from build123d import *
from build123d.topology import SkipClean

# Parameters (mm, degrees)
SKETCH2_R               = 50.165
BOSS_EXTRUDE1_DEPTH     = 38.862
SKETCH3_R               = 14.986
BOSS_EXTRUDE2_DEPTH     = 3.556
BOSS_EXTRUDE3_START     = 2.54
SKETCH4_R               = 50.165
SKETCH4_R_2             = 43.18
BOSS_EXTRUDE3_DEPTH     = 2.54
SKETCH5_R               = 8.89
CUT_EXTRUDE1_DEPTH      = 81.890725637
CIRPATTERN1_COUNT       = 4
CUT_EXTRUDE2_DEPTH      = 83.657977074
CUT_EXTRUDE2_DEPTH_BACK = 83.657977074
SKETCH6_R               = 2.54
SKETCH7_R               = 10.033
SKETCH7_R_2             = 8.001
BOSS_EXTRUDE4_DEPTH     = 1.016
SKETCH8_R               = 4.953
SKETCH8_R_2             = 2.54
BOSS_EXTRUDE5_DEPTH     = 1.016
CHAMFER1_SIZE           = 0.254
FILLET1_R               = 0.254
CHAMFER2_SIZE           = 1.27
CHAMFER3_SIZE           = 1.27
CHAMFER4_SIZE           = 0.254


with BuildPart() as part:
    # Sketch2 → Boss-Extrude1 (new body)
    with BuildSketch(Plane.XY):
        with Locations(Location((0, 0, 0), (0, 0, 180))):
            Circle(SKETCH2_R)
    extrude(amount=BOSS_EXTRUDE1_DEPTH)

    # Sketch3 → Boss-Extrude2 (add)
    with BuildSketch(Plane(origin=(0, 0, 0), x_dir=(-1, 0, 0), z_dir=(0, 0, -1))):
        with Locations(Location((0, 0, 0), (0, 0, 180))):
            Circle(SKETCH3_R)
    boss_extrude2 = extrude(amount=BOSS_EXTRUDE2_DEPTH)

    # Sketch4 → Boss-Extrude3 (add)
    with BuildSketch(Plane(origin=(0, 0, 0), x_dir=(-1, 0, 0), z_dir=(0, 0, -1)).offset(BOSS_EXTRUDE3_START)):
        Circle(SKETCH4_R)
        Circle(SKETCH4_R_2, mode=Mode.SUBTRACT)
    boss_extrude3 = extrude(amount=-BOSS_EXTRUDE3_DEPTH)

    # Sketch5 → Cut-Extrude1 (cut, through all)
    with BuildSketch(Plane(origin=(0, 0, 0), x_dir=(-1, 0, 0), z_dir=(0, 0, -1))):
        with Locations((31.75, 0)):
            Circle(SKETCH5_R)
    cut_extrude1 = extrude(amount=-CUT_EXTRUDE1_DEPTH, mode=Mode.SUBTRACT)

    # CirPattern1: Cut-Extrude1 ×4 about axis
    cirpattern1_axis = Axis((0, 0, 0), (0, 0, 1))
    for i in range(1, CIRPATTERN1_COUNT):
        add(cut_extrude1.rotate(cirpattern1_axis, i * 360 / CIRPATTERN1_COUNT), mode=Mode.SUBTRACT)

    # Mirror1: Boss-Extrude3 across plane
    add(boss_extrude3.mirror(Plane(origin=(0, 0, 19.431), x_dir=(1, 0, 0), z_dir=(0, 0, -1))))

    # Mirror2: Boss-Extrude2 across plane
    add(boss_extrude2.mirror(Plane(origin=(0, 0, 19.431), x_dir=(1, 0, 0), z_dir=(0, 0, -1))))

    # Sketch6 → Cut-Extrude2 (cut, two sides: drawn at the far end of the back side and taken through both)
    with BuildSketch(Plane.XY.offset(-CUT_EXTRUDE2_DEPTH_BACK)):
        Circle(SKETCH6_R)
    extrude(amount=CUT_EXTRUDE2_DEPTH + CUT_EXTRUDE2_DEPTH_BACK, mode=Mode.SUBTRACT)

    # Sketch7 → Boss-Extrude4 (add)
    with BuildSketch(Plane(origin=(0, 0, -3.556), x_dir=(-1, 0, 0), z_dir=(0, 0, -1))):
        Circle(SKETCH7_R)
        Circle(SKETCH7_R_2, mode=Mode.SUBTRACT)
    boss_extrude4 = extrude(amount=BOSS_EXTRUDE4_DEPTH)

    # Sketch8 → Boss-Extrude5 (add)
    with SkipClean():  # the faces are left unmerged after this step: merging them gives an invalid solid
        with BuildSketch(Plane(origin=(0, 0, -3.556), x_dir=(-1, 0, 0), z_dir=(0, 0, -1))):
            Circle(SKETCH8_R)
            Circle(SKETCH8_R_2, mode=Mode.SUBTRACT)
        boss_extrude5 = extrude(amount=BOSS_EXTRUDE5_DEPTH)

    # Chamfer1
    chamfer1_edges = [part.edges().sort_by_distance(p)[0] for p in [
        (10.033, 0, -3.556),
        (8.001, 0, -4.572),
    ]]
    chamfer(chamfer1_edges, length=CHAMFER1_SIZE)

    # Fillet1
    fillet1_edges = [part.edges().sort_by_distance(p)[0] for p in [
        (4.953, 0, -4.572),
        (2.54, 0, -4.572),
    ]]
    fillet(fillet1_edges, radius=FILLET1_R)

    # Chamfer2
    chamfer2_edges = [part.edges().sort_by_distance(p)[0] for p in [
        (-22.86, 0, 38.862),
        (-22.86, 0, 0),
        (0, 22.86, 38.862),
        (0, 22.86, 0),
        (22.86, 0, 38.862),
        (22.86, 0, 0),
        (0, -22.86, 38.862),
        (0, -22.86, 0),
    ]]
    chamfer(chamfer2_edges, length=CHAMFER2_SIZE)

    # Chamfer3
    chamfer3_edges = [part.edges().sort_by_distance(p)[0] for p in [
        (50.165, 0, -2.54),
        (50.165, 0, 41.402),
    ]]
    chamfer(chamfer3_edges, length=CHAMFER3_SIZE)

    # Sketch9 → Cut-Revolve1 (revolve, cut)
    with SkipClean():  # the faces are left unmerged after this step: merging them gives an invalid solid
        with BuildSketch(Plane(origin=(0, 0, 0), x_dir=(0, 0, -1), z_dir=(1, 0, 0)), mode=Mode.PRIVATE) as cut_revolve1_sk:
            Polygon((-5.461, 42.545), (-33.401, 42.545), (-37.211, 50.165), (-1.651, 50.165), align=None)
        revolve(cut_revolve1_sk.sketch.rotate(Axis((0, 0, 38.862), (0, 0, -1)), 270), axis=Axis((0, 0, 38.862), (0, 0, -1)), mode=Mode.SUBTRACT)

    # Mirror3: Boss-Extrude5 across plane
    add(boss_extrude5.mirror(Plane(origin=(0, 0, 19.431), x_dir=(1, 0, 0), z_dir=(0, 0, -1))))

    # Mirror4: Boss-Extrude4 across plane
    add(boss_extrude4.mirror(Plane(origin=(0, 0, 19.431), x_dir=(1, 0, 0), z_dir=(0, 0, -1))))

    # Chamfer4
    chamfer4_edges = [part.edges().sort_by_distance(p)[0] for p in [
        (4.953, 0, 43.434),
        (2.54, 0, 43.434),
        (10.033, 0, 43.434),
        (8.001, 0, 42.418),
    ]]
    chamfer(chamfer4_edges, length=CHAMFER4_SIZE)


solid = part.part
Could you check a few things on this model? Use its own coordinates, in mm. A direction names the side the tool comes from. Give positions to 0.01 mm unless a question says otherwise; leave off trailing zeros. Write each loop counter-clockwise with the first axis right and the second up, starting at its lowest first coordinate (ties: lowest second). Pieces come first, ordered by that corner, then holes. Notation, with made-up numbers: (-18, 7.5) -> (40, 7.5) arc R12 cw to (40, 27.5) -> close; hole circle Ø6 at (19, 61.5). An arc over 180 degrees is marked (long way). Answer as CSV lines item,"result". Start each with the question number.
(1) If we section it at C-C, the plane z = 35.5: Write out the boundary of the cut face in (x, y), and give its area (3 significant figures).
(2) Which directions (+Z, -Z, +X, -X, +Y, -Y) give clear straight access to the entire face, cutting with the end or side of a thin tool? Please do faces 4 (the face through (0, -3, 43.434)), 5 (the face through (-19, -1, 0)), 6 (the face through (31.83, 29.18, 40.15)).
(3) If we section it at B-B, the plane x = 0: Give the number of separate pieces and of enclosed holes in the cut face, and give its area (3 significant figures).
(4) I'm going to push flat-ended pins straight in: pin 1 Ø4 at (x, y) = (6, 23.5) entering from +Z; pin 2 Ø10.5 at (x, y) = (-31.75, 0) entering from +Z; pin 3 Ø3 at (x, y) = (-18.5, -24) entering from -Z; pin 4 Ø2 at (y, z) = (-3.5, 32.5) entering from +X. Where does each tip first touch, or does it pass through?
(5) If we section it at A-A, the plane z = 8: Write out the boundary of the cut face in (x, y) (3 decimals), and give its area (3 significant figures).
(6) If we mould it in two halves opening along Y, with no side actions, what happens to faces 1 (the face through (7.5, 3.8, -4.572)), 2 (the face through (-0.1, 5.2, -3.556)), 3 (the face through (6.53, 49.74, 38.69))? For each: +Y half, -Y half, draft (parallel to the pull), parting line (faces both ways), or undercut.
(7) Please list where these lines run through material, in increasing order: line 1 (Y direction, x = 0, z = -3); line 2 (X direction, y = 3, z = 8); line 3 (X direction, y = -1, z = 41).
Answer list:
1,outline,"circle Ø93.49 at (0, 0); hole circle Ø17.78 at (-31.75, 0); hole circle Ø17.78 at (0, -31.75); hole circle Ø17.78 at (0, 31.75); hole circle Ø5.08 at (0, 0); hole circle Ø17.78 at (31.75, 0)"
1,area,"5,850 mm^2"
2,face 4,"+Z, +X, -X, +Y, -Y"
2,face 5,"-Z"
2,face 6,"+Z"
3,separate pieces,"4"
3,enclosed holes,"0"
3,area,"2,090 mm^2"
4,pin 1,"z = 38.86"
4,pin 2,"through"
4,pin 3,"z = 0"
4,pin 4,"x = 42.6"
5,outline,"circle Ø85.09 at (0, 0); hole circle Ø17.78 at (-31.75, 0); hole circle Ø17.78 at (0, -31.75); hole circle Ø17.78 at (0, 31.75); hole circle Ø5.08 at (0, 0); hole circle Ø17.78 at (31.75, 0)"
5,area,"4,670 mm^2"
6,face 1,"draft"
6,face 2,"undercut"
6,face 3,"parting line"
7,line 1,"-14.99 to -2.54, 2.54 to 14.99"
7,line 2,"-42.44 to -40.12, -23.38 to 23.38, 40.12 to 42.44"
7,line 3,"-49.29 to -43.17, -14.95 to -2.33, 2.33 to 14.95, 43.17 to 49.29"
